Part model, mm, in its own coordinate system. A direction names the side the tool comes from. Round coordinates to 2 decimals unless told otherwise and drop trailing zeros. Write each loop counter-clockwise with the first axis right and the second up, starting at its lowest first coordinate (ties: lowest second). Pieces come first, ordered by that corner, then holes. Notation, with made-up numbers: M -23.75,46.5 L 34.25,46.5 A27 ccw 34.25,65.5 Z; hole C 11,-15.75 d2. An arc over 180 degrees is marked long. Answer as a JSON object with one key per item and string values. Group by question number.
1. Band-saw the part on A-A, the plane z = 700.5. Write the cut outline in (x, y) (3 decimals), plus the area to 3 significant figures.
2. Drop flat-ended pins along their axis: pin 1 (9.5 mm diameter, centred on x = 22.225, z = 762, fed in from +Y) (3 decimals); pin 2 (8 mm diameter, centred on y = 18.26, z = 31.75, fed in from +X) (3 decimals). Give the stop position or say it passes through.
3. Drill centre lines: line 1 (Z direction, x = 3, y = 17); line 2 (X direction, y = 18.5, z = 444) (3 decimals). Where is each one in solid material? Low to high. Write a range as from..to.
4. Which spindle directions (+Z, -Z, +X, -X, +Y, -Y) get a long thin tool onto all of the face, cutting with end or side? Do faces 1 (the face through (34.48, 1.61, 3.82)), 2 (the face through (22, 3.175, 394)). Say none if no direction does.
from build123d import *

# Parameters (mm, degrees)
BASE_FLANGE1_DEPTH              = 800.1
FILLET1_R                       = 12.7
F_9_32_0_28125_DIAMETER_HOLE1_D = 7.14375
F_9_32_0_28125_DIAMETER_HOLE2_D = 7.14375


# Sheet-metal steps are written as plain solids
with BuildPart() as part:
    # Sketch1 → Base-Flange1 (new body)
    with BuildSketch(Plane.XY):
        with BuildLine():
            Line((0, 38.1), (0, 6.35))
            ThreePointArc((0, 6.35), (1.859871939, 1.859871939), (6.35, 0))
            Line((6.35, 0), (38.1, 0))
            Line((38.1, 0), (38.1, 3.175))
            Line((38.1, 3.175), (6.35, 3.175))
            ThreePointArc((6.35, 3.175), (4.10493597, 4.10493597), (3.175, 6.35))
            Line((3.175, 6.35), (3.175, 38.1))
            Line((3.175, 38.1), (0, 38.1))
        make_face()
    extrude(amount=BASE_FLANGE1_DEPTH)

    # Fillet1
    fillet1_edges = [part.edges().sort_by_distance(p)[0] for p in [
        (1.5875, 38.1, 800.1),
        (1.5875, 38.1, 0),
        (38.1, 1.5875, 800.1),
        (38.1, 1.5875, 0),
    ]]
    fillet(fillet1_edges, radius=FILLET1_R)

    # 9/32 (0.28125) Diameter Hole1 (through all)
    with Locations(Plane(origin=(3.175, 0, 0), x_dir=(0, 0, -1), z_dir=(1, 0, 0))):
        with Locations((-768.35, 18.25625), (-514.35, 18.25625), (-285.75, 18.25625), (-31.75, 18.25625)):
            Hole(F_9_32_0_28125_DIAMETER_HOLE1_D / 2)

    # 9/32 (0.28125) Diameter Hole2 (through all)
    with Locations(Plane(origin=(0, 3.175, 0), x_dir=(1, 0, 0), z_dir=(0, 1, 0))):
        with Locations((22.225, -38.1), (22.225, -762)):
            Hole(F_9_32_0_28125_DIAMETER_HOLE2_D / 2)


solid = part.part
Worked answers:
{
 "1": {"outline": "M 0,6.35 A6.35 ccw 6.35,0 L 38.1,0 L 38.1,3.175 L 6.35,3.175 A3.175 cw 3.175,6.35 L 3.175,38.1 L 0,38.1 Z", "area": "225 mm^2"},
 "2": {"pin 1": "stops at y = 3.175", "pin 2": "stops at x = 3.175"},
 "3": {"line 1": "z = 0..28.41, 35.09..282.41, 289.09..511.01, 517.69..765.01, 771.69..800.1", "line 2": "x = 0..3.175"},
 "4": {"face 1": "-Z, +X, +Y, -Y", "face 2": "+Z, -Z, +X, +Y"}
}
